Autodesk Inventor part; units mm, degrees
ref_plane "Plano de trabajo1" through (-5, 393, 0) normal (0, 1, 0) x (-1, 0, 0)
ref_plane "YZ Plane" through (0, 0, 0) normal (1, 0, 0) x (0, 1, 0)
ref_plane "XY Plane" through (0, 0, 0) normal (0, 0, 1) x (1, 0, 0)
sketch "Boceto1" plane through (0, 0, 0) normal (0, 0, 1) x (1, 0, 0)
  line L0 (0, 0) -> (-3, 0)
  arc A0 (-5, 2) -> (-3, 0) centre (-3, 2) ccw
  line L1 (-5, 2) -> (-5, 393)
  dimension "d0" = 391
  dimension "d1" = 2
  dimension "d2" = 5
ref_plane "Plano de trabajo1" through (-5, 393, 0) normal (0, 1, 0) x (-1, 0, 0)
sketch "Boceto2" plane through (-5, 393, 0) normal (0, 1, 0) x (-1, 0, 0)
  circle A0 centre (0, 0) radius 1.25
  point P0 (-5, 0)
  point P1 (0, 0)
  point P2 (0, 0)
  point P3 (0, 0)
  dimension "d3" = 2.5
sweep "Barrido1" add profiles "Boceto2" path "Boceto1"
sketch "Boceto4" plane through (0, 0, 0) normal (1, 0, 0) x (0, 0, -1)
  point P0 (0, 0)
  point P1 (0, 0)
sketch "Boceto3" plane through (0, 0, 0) normal (1, 0, 0) x (0, 0, -1)
  circle A0 centre (0, 0) radius 2
  point P0 (0, 0)
  dimension "d6" = 4
extrude "Extrusión1" add sketch "Boceto3" along normal blind 0.5
fillet "Empalme1" radius 0.25 1 edges at (0, 1.25, 0)
fillet "Empalme2" radius 0.25 2 edges at (0, 0, 2) (0.5, 0, 2)
thread "Rosca1"
properties part number "radio" material "Acero inoxidable"
Here's how the part is built. I have some questions about the finished solid (model axes, mm). Coordinates: 2 decimals unless noted, no trailing zeros. Order: outer loops, then holes, each group sorted by start corner. A loop starts at its lowest first (then second) coordinate and runs counter-clockwise, first axis right, second up. Notation, with made-up numbers: (-9, 26.5) - (19, 26.5) arc R36 cw to (19, 65.5) - close; hole circle Ø10 at (-23, 49). An arc over 180 degrees is marked (long way). One line per question, with ' | ' between items.
(1) Will these pins go through, and if not, where does the flat tip stop? pin 1 (1.8 mm diameter, centred on y = 0.5, z = -0.5, fed in from -X); pin 2 (1.5 mm diameter, centred on y = 72.5, z = 1, fed in from +X).
Report:
pin 1: stops at x = -6.17 | pin 2: stops at x = -3.78
(2) Suppose I cut it at B-B on x = -1.75. List the corners of the cut face in (y, z) for me, and give its area (3 significant figures).
Report:
outline: circle Ø2.5 at (0, 0) | area: 4.91 mm2
(3) Suppose I cut it at C-C on y = 131.5. List the corners of the cut face in (x, z) for me, and give its area (3 significant figures).
Report:
outline: circle Ø2.5 at (-5, 0) | area: 4.91 mm2
(4) If I drill on L1, parallel to Y at x = -0.25, z = 0.15; L2, parallel to X at y = 305.5, z = 0; L3, parallel to Y at x = -5, z = 1.05, over which ranges is the centre line in solid material (lowest first)?
Report:
L1: y = -1.24 to 1.24 | L2: x = -6.25 to -3.75 | L3: y = 0.22 to 393
